Part model, mm, in its own coordinate system. A direction names the side the tool comes from. Give positions to 0.01 mm unless a question says otherwise; leave off trailing zeros. Order: outer loops, then holes, each group sorted by start corner. A loop starts at its lowest first (then second) coordinate and runs counter-clockwise, first axis right, second up. Notation, with made-up numbers: M 38,0.25 L 49,0.25 A4 cw 49,6.25 Z; hole C 80,7 d10. An arc over 180 degrees is marked long. Return JSON: item names as keys, results as strings.
from build123d import *

# Parameters (mm, degrees)
EXTRUDE_START               = -443
EXTRUDE_1_DEPTH             = 10
EXTRUDE_START_2             = -345
EXTRUDE_1_2_OUTLINE_W       = 17
EXTRUDE_1_2_OUTLINE_H       = 4.342105263
EXTRUDE_1_2_DEPTH           = 8.417172155
EXTRUDE_2_DEPTH             = 28
EXTRUDE_3_DEPTH             = 1.157894737
EXTRUDE_4_DEPTH             = 4
SKETCH_5_W                  = 4
SKETCH_5_H                  = 45
EXTRUDE_5_DEPTH             = 13
EXTRUDE_6_DEPTH             = 5
THICKEN_START               = -471
THICKEN_1_DEPTH             = 4
SKETCH_7_W                  = 13
SKETCH_7_H                  = 7
CUT_EXTRUDE_1_DEPTH         = 65.235893393
SKETCH_8_W                  = 2
SKETCH_8_H                  = 3
CUT_EXTRUDE_2_DEPTH         = 65.235893393
SKETCH_9_W                  = 2
SKETCH_9_H                  = 3
CUT_EXTRUDE_3_DEPTH         = 65.235893393
CUT_EXTRUDE_4_DEPTH         = 475.157146946
CUT_EXTRUDE_5_DEPTH         = 475.157146946
SKETCH_12_W                 = 16.5
SKETCH_12_H                 = 15.5
CUT_EXTRUDE_6_DEPTH         = 474.337353269
CUT_EXTRUDE_7_DEPTH         = 1
CUT_EXTRUDE_8_DEPTH         = 1
CUT_EXTRUDE_9_DEPTH         = 1
HOLE_WIZARD_3_6_3_6_1_D     = 3.6
HOLE_WIZARD_3_6_3_6_1_DEPTH = 50
CHAMFER_1_SIZE              = 2
FILLET_1_R                  = 10


with BuildPart() as part:
    # 凸台-拉伸1: read off the stored shape, not the designer's step
    # 凸台-拉伸1 outline → 凸台-拉伸1 (new body)
    with BuildSketch(Plane.YZ.offset(EXTRUDE_START)):
        Polygon((-10.657894737, 43), (-13.5, 31), (-13.5, 5), (-10.657894737, 5), align=None)
    extrude(amount=EXTRUDE_1_DEPTH)

    # Extrude 1 2 outline → Extrude 1 2 (cut)
    with BuildSketch(Plane(origin=(0, 0, 0), x_dir=(0.707106781186548, 0, 0.707106781186547), z_dir=(0.707106781186547, 0, -0.707106781186548)).offset(EXTRUDE_START_2)):
        with Locations((-282.5, 12.828947369)):
            Rectangle(EXTRUDE_1_2_OUTLINE_W, EXTRUDE_1_2_OUTLINE_H)
    extrude(amount=EXTRUDE_1_2_DEPTH, mode=Mode.SUBTRACT)

    # 草图2 → 凸台-拉伸2 (add)
    with BuildSketch(Plane.ZY.offset(443)):
        Polygon((5, -10.657894737), (33, -10.657894737), (33, -13.026315789), (31, -13.5), (5, -13.5), align=None)
    extrude(amount=EXTRUDE_2_DEPTH)

    # 草图3 → 凸台-拉伸3 (add)
    with BuildSketch(Plane(origin=(0, -10.657894737, 0), x_dir=(-1, 0, 0), z_dir=(0, 1, 0))):
        Polygon((471, 5), (433, 5), (433, 43), (443, 33), (471, 33), align=None)
    extrude(amount=EXTRUDE_3_DEPTH)

    # 草图4 → 凸台-拉伸4 (add)
    with BuildSketch(Plane(origin=(-433, 0, 0), x_dir=(0, 0, -1), z_dir=(1, 0, 0))):
        Polygon((-50, -9), (-5, -9), (-5, -13.5), (-31, -13.5), align=None)
    extrude(amount=EXTRUDE_4_DEPTH)

    # 草图5 → 凸台-拉伸5 (add)
    with BuildSketch(Plane(origin=(0, -9, 0), x_dir=(-1, 0, 0), z_dir=(0, 1, 0))):
        with Locations((431, 27.5)):
            Rectangle(SKETCH_5_W, SKETCH_5_H)
    extrude(amount=EXTRUDE_5_DEPTH)

    # 草图6 → 凸台-拉伸6 (add)
    with BuildSketch(Plane(origin=(0, 0, 5), x_dir=(-1, 0, 0), z_dir=(0, 0, -1))):
        with BuildLine():
            Line((429, -13.5), (429, 7.771887242))
            ThreePointArc((429, 7.771887242), (450, 12.5), (471, 7.771887242))
            Line((471, 7.771887242), (471, -13.5))
            Line((471, -13.5), (429, -13.5))
        make_face()
    extrude(amount=EXTRUDE_6_DEPTH)

    # 加厚1: read off the stored shape, not the designer's step
    # 加厚1 outline → 加厚1 (add)
    with BuildSketch(Plane.YZ.offset(THICKEN_START)):
        Polygon((2, 5), (-9.5, 16.5), (-9.5, 5), align=None)
    extrude(amount=THICKEN_1_DEPTH)

    # 草图7 → 切除-拉伸1 (cut, through all)
    with BuildSketch(Plane.ZY.offset(433)):
        with Locations((32.5, -2.5)):
            Rectangle(SKETCH_7_W, SKETCH_7_H)
    extrude(amount=-CUT_EXTRUDE_1_DEPTH, mode=Mode.SUBTRACT)

    # 草图8 → 切除-拉伸2 (cut, through all)
    with BuildSketch(Plane.ZY.offset(433)):
        with Locations((46, 0.5)):
            Rectangle(SKETCH_8_W, SKETCH_8_H)
    extrude(amount=-CUT_EXTRUDE_2_DEPTH, mode=Mode.SUBTRACT)

    # 草图9 → 切除-拉伸3 (cut, through all)
    with BuildSketch(Plane.ZY.offset(433)):
        with Locations((46, -5.5)):
            Rectangle(SKETCH_9_W, SKETCH_9_H)
    extrude(amount=-CUT_EXTRUDE_3_DEPTH, mode=Mode.SUBTRACT)

    # 草图10 → 切除-拉伸4 (cut, through all)
    with BuildSketch(Plane(origin=(0, -9.5, 0), x_dir=(-1, 0, 0), z_dir=(0, 1, 0))):
        with BuildLine():
            Line((438.3, 29.000393674), (438.3, 10.000393674))
            ThreePointArc((438.3, 10.000393674), (440, 8.300393674), (441.7, 10.000393674))
            Line((441.7, 10.000393674), (441.7, 29.000393674))
            ThreePointArc((441.7, 29.000393674), (440, 30.700393674), (438.3, 29.000393674))
        make_face()
    extrude(amount=-CUT_EXTRUDE_4_DEPTH, mode=Mode.SUBTRACT)

    # 草图11 → 切除-拉伸5 (cut, through all)
    with BuildSketch(Plane(origin=(0, -9.5, 0), x_dir=(-1, 0, 0), z_dir=(0, 1, 0))):
        with BuildLine():
            Line((458.3, 29.000393674), (458.3, 17.000393674))
            ThreePointArc((458.3, 17.000393674), (460, 15.300393674), (461.7, 17.000393674))
            Line((461.7, 17.000393674), (461.7, 29.000393674))
            ThreePointArc((461.7, 29.000393674), (460, 30.700393674), (458.3, 29.000393674))
        make_face()
    extrude(amount=-CUT_EXTRUDE_5_DEPTH, mode=Mode.SUBTRACT)

    # 草图12 → 切除-拉伸6 (cut, through all)
    with BuildSketch(Plane.XY.offset(5)):
        with Locations((-450, 0)):
            Rectangle(SKETCH_12_W, SKETCH_12_H)
    extrude(amount=-CUT_EXTRUDE_6_DEPTH, mode=Mode.SUBTRACT)

    # 草图13 → 切除-拉伸7 (cut)
    with BuildSketch(Plane.XY.offset(5)):
        Polygon((-458.25, 1.385640646), (-459.125, 2.901185103), (-462.475, 2.901185103), (-464.15, 0), (-462.475, -2.901185103), (-459.125, -2.901185103), (-458.25, -1.385640646), align=None)
    extrude(amount=-CUT_EXTRUDE_7_DEPTH, mode=Mode.SUBTRACT)

    # 草图14 → 切除-拉伸8 (cut)
    with BuildSketch(Plane.XY.offset(5)):
        Polygon((-441.75, 2.414359354), (-440.875, 0.898814897), (-437.525, 0.898814897), (-435.85, 3.8), (-437.525, 6.701185103), (-440.875, 6.701185103), (-441.75, 5.185640646), align=None)
    extrude(amount=-CUT_EXTRUDE_8_DEPTH, mode=Mode.SUBTRACT)

    # 草图15 → 切除-拉伸9 (cut)
    with BuildSketch(Plane.XY.offset(5)):
        Polygon((-441.75, -5.185640646), (-440.875, -6.701185103), (-437.525, -6.701185103), (-435.85, -3.8), (-437.525, -0.898814897), (-440.875, -0.898814897), (-441.75, -2.414359354), align=None)
    extrude(amount=-CUT_EXTRUDE_9_DEPTH, mode=Mode.SUBTRACT)

    # Ø3.6 (3.6) 直径孔1
    with Locations(Plane(origin=(0, 0, 0), x_dir=(-1, 0, 0), z_dir=(0, 0, -1))):
        with Locations((439.2, -3.8), (439.2, 3.8), (460.8, 0)):
            Hole(HOLE_WIZARD_3_6_3_6_1_D / 2, depth=HOLE_WIZARD_3_6_3_6_1_DEPTH)

    # 倒角1
    chamfer_1_edges = [part.edges().sort_by_distance(p)[0] for p in [
        (-431, 4, 5),
        (-441.75, -7.75, 2.5),
        (-458.25, -7.75, 2.5),
    ]]
    chamfer(chamfer_1_edges, length=CHAMFER_1_SIZE)

    # 圆角1
    fillet_1_edges = [part.edges().sort_by_distance(p)[0] for p in [
        (-443, -11.842105263, 33),
        (-433, -10.078947368, 43),
    ]]
    fillet(fillet_1_edges, radius=FILLET_1_R)


solid = part.part
Q1. 3-axis set-ups, long thin cutter, end or side, ignore diameter. For faces 5 (the flat face through (-431, -6, 45)), 6 (the flat face through (-436.676, -2.37, 4.507)), 7 (the cylindrical face through (-460, -11.5, 15.3)), 8 (the flat face through (-450, 7.75, 3)): which of +Z, -Z, +X, -X, +Y, -Y reach the whole face in a straight line?
Established:
{"face 5": "+X, -X", "face 6": "+Z", "face 7": "+Y, -Y", "face 8": "+Z, -Z"}
Q2. Pin check, flat tips, straight feed: pin 1 (12 mm diameter, centred on x = -456, y = -4, fed in from +Z); pin 2 (2 mm diameter, centred on x = -430.5, z = 45.5, fed in from +Y); pin 3 (4.5 mm diameter, centred on x = -439.2, y = -3.8, fed in from -Z); pin 4 (4.5 mm diameter, centred on x = -440, y = 3.5, fed in from +Z). Stop position of each tip, or through.
Established:
{"pin 1": "stops at z = 33", "pin 2": "stops at y = 4", "pin 3": "stops at z = 0", "pin 4": "stops at z = 5"}
Q3. Two-plate mould, pull along Z, no slides. Class faces 1 (the flat face through (-438.3, -11, 20)), 2 (the flat face through (-436.7, 2.33, 4.51)), 3 (the flat face through (-458.3, -11, 23)), 4 (the flat face through (-450, -9, 0)): +Z half, -Z half, draft (parallel to the pull), parting line (faces both ways), or undercut.
Established:
{"face 1": "undercut", "face 2": "draft", "face 3": "undercut", "face 4": "-Z half"}
Q4. Band-saw the part on B-B (x = -461). Give the cut face in (y, z), then the cut area to 3 significant figures.
Established:
{"outline": "M -13.5,0 L -1.79,0 L -1.79,4 L -2.9,4 L -2.9,5 L -9.5,5 L -9.5,15.63 L -13.5,15.63 Z; M -13.5,30.38 L -9.5,30.38 L -9.5,33 L -13.03,33 L -13.5,31 Z; M 1.79,0 L 11.25,0 L 11.25,5 L 2.9,5 L 2.9,4 L 1.79,4 Z", "area": "156 mm²"}
Q5. Band-saw the part on A-A (z = 12). Give the cut face in (x, y).
Established:
{"outline": "M -471,-13.5 L -441.7,-13.5 L -441.7,-9.5 L -467,-9.5 L -467,-5 L -471,-5 Z; M -438.3,-13.5 L -429,-13.5 L -429,4 L -433,4 L -433,-9.5 L -438.3,-9.5 Z"}
Q6. Probe line 1 along Z through (x, y) = (-432.5, 0.25); line 2 along Y through (x, z) = (-439, 1); line 3 along Y through (x, z) = (-439.2, 2.4). List the from-to ranges inside material, lowest first.
Established:
{"line 1": "z = 0 to 26, 39 to 45, 47 to 50", "line 2": "y = -13.5 to -5.59, -2.01 to 2.01, 5.59 to 11.25", "line 3": "y = -13.5 to -5.6, -2 to 2, 5.6 to 11.29"}
Q7. Band-saw the part on D-D (x = -445). Give the cut face in (y, z), then the cut area to 3 significant figures.
Established:
{"outline": "M -13.5,0 L -7.75,0 L -7.75,5 L -9.5,5 L -9.5,33.23 L -12.97,33.23 L -13.5,31 Z; M 7.75,0 L 12.24,0 L 12.24,5 L 7.75,5 Z", "area": "164 mm²"}
Q8. Band-saw the part on C-C (z = 18). Give the cut face in (x, y), then the cut area to 3 significant figures.
Established:
{"outline": "M -471,-13.5 L -461.7,-13.5 L -461.7,-9.5 L -471,-9.5 Z; M -458.3,-13.5 L -441.7,-13.5 L -441.7,-9.5 L -458.3,-9.5 Z; M -438.3,-13.5 L -429,-13.5 L -429,4 L -433,4 L -433,-9.5 L -438.3,-9.5 Z", "area": "195 mm²"}
